Study the drawing (mm; zero at the part's minimum x, y, z) and answer. Round coordinates to 2 decimals unless told otherwise and drop trailing zeros. Order: outer loops, then holes, each group sorted by start corner. A loop starts at its lowest first (then second) coordinate and runs counter-clockwise, first axis right, second up. Notation, with made-up numbers: (26, -19) - (79, -19) arc R27 cw to (79, 11) - close; hole circle Ø11 at (-31, 18). An arc over 180 degrees is marked (long way). Put each result on its own line as item: value.
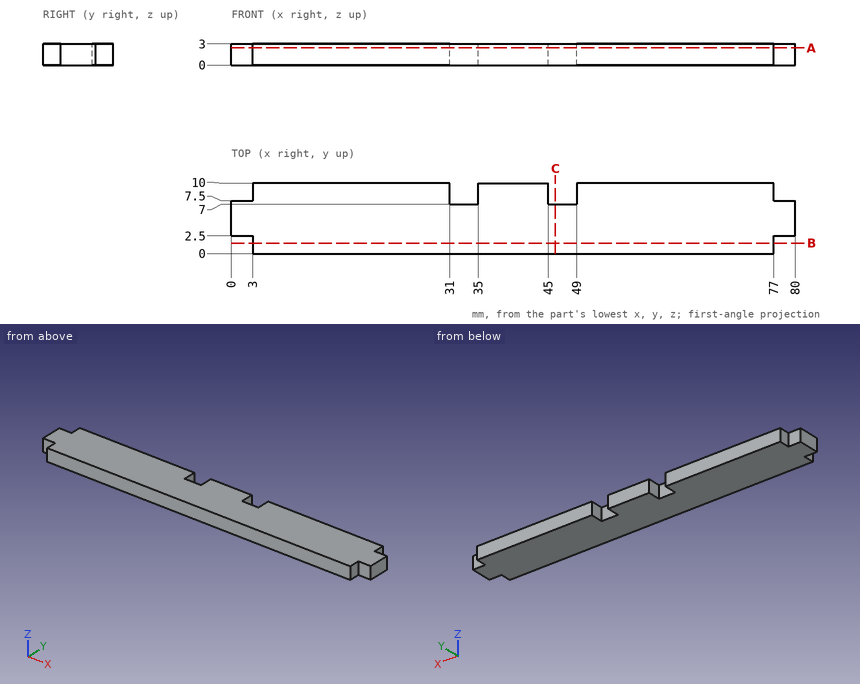
1) Straight lines are drawn through the part: L1, parallel to X at y = 9.75, z = 1.65; L2, parallel to X at y = 2, z = 1.85; L3, parallel to Y at x = 48, z = 1.9. For each, find the intervals that lie inside material, in ascending order. Write a range as from..to.
Findings below:
L1: x = 3..31, 35..45, 49..77
L2: x = 3..77
L3: y = 0..7
2) A cutting plane is placed at B-B on y = 1.5. Write down the section's boundary in (x, z).
Findings below:
outline: (3, 0) - (77, 0) - (77, 3) - (3, 3) - close
3) A cutting plane is placed at C-C on x = 46. Write down the section's boundary in (y, z), then the cut area to 3 significant figures.
Findings below:
outline: (0, 0) - (7, 0) - (7, 3) - (0, 3) - close
area: 21.0 mm2
4) Given pin 1 Ø0.9 at (x, z) = (2, 2) entering from +Y; pin 2 Ø1.5 at (x, z) = (1, 1.5) entering from -Y; pin 3 Ø0.9 at (y, z) = (8, 2) entering from +X, each flat-ended and moving along its own axis, determine where each tip first touches the part or whether it passes through.
Findings below:
pin 1: stops at y = 7.5
pin 2: stops at y = 2.5
pin 3: stops at x = 77
5) A cutting plane is placed at A-A on z = 2.45. Write down the section's boundary in (x, y), then the cut area to 3 significant figures.
Findings below:
outline: (0, 2.5) - (3, 2.5) - (3, 0) - (77, 0) - (77, 2.5) - (80, 2.5) - (80, 7.5) - (77, 7.5) - (77, 10) - (49, 10) - (49, 7) - (45, 7) - (45, 10) - (35, 10) - (35, 7) - (31, 7) - (31, 10) - (3, 10) - (3, 7.5) - (0, 7.5) - close
area: 746 mm2
